Geometry check sheet. Reference: the model listing, model coordinates, mm. A direction names the side the tool comes from. Coordinates: 2 decimals unless noted, no trailing zeros. Write each loop counter-clockwise with the first axis right and the second up, starting at its lowest first coordinate (ties: lowest second). Pieces come first, ordered by that corner, then holes. Notation, with made-up numbers: (-30, 67.25) - (1, 67.25) arc R29 ccw to (1, 94.25) - close; hole circle Ø2 at (75, 54.5). An arc over 180 degrees is marked (long way). Answer as a JSON object with one key per item and string values. Group by question number.
from build123d import *

# Parameters (mm, degrees)
SKETCH_W        = 30
SKETCH_H        = 40
PAD_DEPTH       = 40
SKETCH001_W     = 20
SKETCH001_H     = 70
POCKET_DEPTH    = 25
SKETCH002_W     = 18
SKETCH002_H     = 62
POCKET001_DEPTH = 5
SKETCH003_R     = 1
POCKET002_DEPTH = 5
SKETCH004_W     = 10
SKETCH004_H     = 10
POCKET003_DEPTH = 5
SKETCH005_W     = 10
SKETCH005_H     = 10
POCKET004_DEPTH = 5
FILLET_R        = 3


with BuildPart() as part:
    # Sketch → Pad (new body, symmetric)
    with BuildSketch(Plane.YZ):
        with Locations((-15, 20)):
            Rectangle(SKETCH_W, SKETCH_H)
    extrude(amount=PAD_DEPTH, both=True)

    # Sketch001 (on Face1 of Pad) → Pocket (cut)
    with BuildSketch(Plane(origin=(0, 0, 40), x_dir=(0, -1, 0), z_dir=(0, 0, 1))):
        with Locations((15, 0)):
            Rectangle(SKETCH001_W, SKETCH001_H)
    extrude(amount=-POCKET_DEPTH, mode=Mode.SUBTRACT)

    # Sketch002 (on Face11 of Pocket) → Pocket001 (cut)
    with BuildSketch(Plane(origin=(0, 0, 15), x_dir=(0, -1, 0), z_dir=(0, 0, 1))):
        with Locations((15, 0)):
            Rectangle(SKETCH002_W, SKETCH002_H)
    extrude(amount=-POCKET001_DEPTH, mode=Mode.SUBTRACT)

    # Sketch003 (on Face11 of Pocket001) → Pocket002 (cut)
    with BuildSketch(Plane(origin=(0, 0, 15), x_dir=(0, -1, 0), z_dir=(0, 0, 1))):
        with Locations((7, 33)):
            Circle(SKETCH003_R)
        with Locations((23, -33)):
            Circle(SKETCH003_R)
    extrude(amount=-POCKET002_DEPTH, mode=Mode.SUBTRACT)

    # Sketch004 (on Face3 of Pocket002) → Pocket003 (cut)
    with BuildSketch(Plane(origin=(-40, 0, 0), x_dir=(0, 1, 0), z_dir=(-1, 0, 0))):
        with Locations((-12, -20)):
            Rectangle(SKETCH004_W, SKETCH004_H)
    extrude(amount=-POCKET003_DEPTH, mode=Mode.SUBTRACT)

    # Sketch005 → Pocket004 (cut)
    with BuildSketch(Plane.YZ.offset(40)):
        with Locations((-18, 20.255899)):
            Rectangle(SKETCH005_W, SKETCH005_H)
    extrude(amount=-POCKET004_DEPTH, mode=Mode.SUBTRACT)

    # Fillet
    fillet_edges = [part.edges().sort_by_distance(p)[0] for p in [
        (40, -30, 20),
        (40, 0, 20),
        (-40, 0, 20),
        (-40, -30, 20),
    ]]
    fillet(fillet_edges, radius=FILLET_R)


solid = part.part
(1) Section check A-A (z = 20). Record the cut outline in (x, y), and give its area (3 significant figures).
(2) Material ranges on L1, parallel to X at y = -7, z = 12.4; L2, parallel to X at y = -23, z = 13.8; L3, parallel to Y at x = 23.5, z = 15.5, recorded low to high. Write a range as [from, to].
(3) Section check B-B (y = -15.25). Record the cut outline in (x, z).
(4) Gauge pin test, flat ends, axial feed: pin 1 (0.6 mm diameter, centred on x = -33, y = -23.5, fed in from +Z); pin 2 (1.5 mm diameter, centred on y = -18.5, z = 17, fed in from +X). Record the tip position at first contact, or that the pin passes through.
(5) Draft check along Y on faces 4 (the face through (1, 0, 20)), 5 (the face through (39.1, -29.14, 20.28)), 6 (the face through (-38, -17, 20)), 7 (the face through (40, -12.5, 20.3)). Enter one of: +Y half, -Y half, draft (parallel to the pull), parting line (faces both ways), or undercut.
(6) Set-up check for faces 1 (the face through (38, -18, 15.256)), 2 (the face through (-38, -7, 20)), 3 (the face through (-35, -15, 30)): record each of +Z, -Z, +X, -X, +Y, -Y from which the full face is reachable in a straight line by a thin tool's end or side.
(7) Section check C-C (x = -33). Record the cut outline in (y, z), and give its area (3 significant figures).
Conclusion:
{
 "1": {"outline": "(-40, -27) arc R3 ccw to (-37, -30) - (37, -30) arc R3 ccw to (40, -27) - (40, -23) - (35, -23) - (35, -25) - (-35, -25) - (-35, -17) - (-40, -17) - close; (-40, -7) - (-35, -7) - (-35, -5) - (35, -5) - (35, -13) - (40, -13) - (40, -3) arc R3 ccw to (37, 0) - (-37, 0) arc R3 ccw to (-40, -3) - close", "area": "892 mm^2"},
 "2": {"L1": "x = [-40, -31], [31, 32], [34, 40]", "L2": "x = [-40, -34], [-32, -31], [31, 40]", "L3": "y = [-30, -25], [-5, 0]"},
 "3": {"outline": "(-40, 0) - (40, 0) - (40, 15.26) - (35, 15.26) - (35, 15) - (31, 15) - (31, 10) - (-31, 10) - (-31, 15) - (-40, 15) - close; (-40, 25) - (-35, 25) - (-35, 40) - (-40, 40) - close; (35, 25.26) - (40, 25.26) - (40, 40) - (35, 40) - close"},
 "4": {"pin 1": "stops at z = 10", "pin 2": "stops at x = -35"},
 "5": {"face 4": "+Y half", "face 5": "-Y half", "face 6": "undercut", "face 7": "draft"},
 "6": {"face 1": "+X", "face 2": "-X", "face 3": "+Z"},
 "7": {"outline": "(-30, 0) - (0, 0) - (0, 40) - (-5, 40) - (-5, 15) - (-22, 15) - (-22, 10) - (-24, 10) - (-24, 15) - (-25, 15) - (-25, 40) - (-30, 40) - close", "area": "690 mm^2"}
}
